Geometry check sheet. Reference: the model listing, model coordinates, mm. A direction names the side the tool comes from. Give positions to 0.01 mm unless a question says otherwise; leave off trailing zeros.
1. Release check for a two-part mould opening along Z. For faces 5 (the flat face through (22, 0, -12)), 6 (the flat face through (24, 0, -22)), 7 (the flat face through (9.6, -0.1, -2)), 8 (the flat face through (90, 0, 1)) record: +Z half, -Z half, draft (parallel to the pull), parting line (faces both ways), or undercut.
2. Go/stop test with flat-tipped pins: pin 1 Ø10 at (x, y) = (11.5, 1.5) entering from +Z; pin 2 Ø0.8 at (x, y) = (2.5, 2) entering from +Z; pin 3 Ø3.5 at (x, y) = (143.5, 0) entering from -Z. Record where each tip stops, or that it passes through.
3. Cross-section at A-A, the plane x = 143.5. State how many separate pieces and enclosed holes the cut face has, plus the area to 3 significant figures.
4. Material ranges on L1, parallel to Y at x = 12, z = -0.8; L2, parallel to Y at x = 38.5, z = 34.8; L3, parallel to X at y = -0.5, z = 17, recorded low to high.
5. Tool access check on faces 1 (the flat face through (2, 0, -18)), 2 (the cylindrical face through (6.254, -9.829, -16.143)), 3 (the cylindrical face through (6.2, -9.83, -7.81)), 4 (the flat face through (90, 0, 32)). Record the directions out of +Z, -Z, +X, -X, +Y, -Y that give a thin tool (end or side, any length) a straight path to the whole face; none if there is none.
from build123d import *

# Parameters (mm, degrees)
SKETCH_W          = 124
SKETCH_H          = 31
PAD_DEPTH         = 10
SKETCH001_R       = 2.1
POCKET_DEPTH      = 33.001
POCKET_DEPTH_BACK = 25.001
SKETCH002_R       = 4.5
POCKET001_DEPTH   = 33.001
FILLET_R          = 2
SKETCH003_R       = 1.6
POCKET002_DEPTH   = 4.001
FILLET001_R       = 0.6


with BuildPart() as part:
    # Sketch → Pad (new body, symmetric)
    with BuildSketch(Plane.XZ):
        Polygon((0, 0), (0, -22), (2, -22), (2, -14.6), (3.5, -14.6), (3.5, -18), (4.5, -18), (8.2, -14.6), (8.2, -9.4), (4.5, -6), (3.5, -6), (3.5, -9.4), (2, -9.4), (2, -2), (22, -2), (22, -22), (27, -22), (157, -5), (157, 0), (157, 36), (25, 36), align=None)
        with Locations((91, 16.5)):
            Rectangle(SKETCH_W, SKETCH_H, mode=Mode.SUBTRACT)
    extrude(amount=PAD_DEPTH, both=True)

    # Sketch001 (on Face14 of Pad) → Pocket (cut, two sides)
    with BuildSketch(Plane(origin=(0, 0, 3), x_dir=(1, 0, 0), z_dir=(0, 0, -1))) as pocket_sk:
        with Locations((12, 0)):
            Circle(SKETCH001_R)
    extrude(amount=-POCKET_DEPTH, mode=Mode.SUBTRACT)
    extrude(pocket_sk.sketch, amount=POCKET_DEPTH_BACK, mode=Mode.SUBTRACT)

    # Sketch002 (on Face14 of Pad) → Pocket001 (cut, through all)
    with BuildSketch(Plane(origin=(0, 0, 3), x_dir=(1, 0, 0), z_dir=(0, 0, -1))):
        with Locations((12, 0)):
            Circle(SKETCH002_R)
    extrude(amount=-POCKET001_DEPTH, mode=Mode.SUBTRACT)

    # Fillet
    fillet_edges = [part.edges().sort_by_distance(p)[0] for p in [
        (7.500022, -0.014101, 10.800032),
    ]]
    fillet(fillet_edges, radius=FILLET_R)

    # Sketch003 (on Face25 of Fillet) → Pocket002 (cut, through all)
    with BuildSketch(Plane(origin=(0, 0, 32), x_dir=(1, 0, 0), z_dir=(0, 0, -1))):
        with Locations((38.5, 0)):
            Circle(SKETCH003_R)
        with Locations((143.5, 0)):
            Circle(SKETCH003_R)
    extrude(amount=-POCKET002_DEPTH, mode=Mode.SUBTRACT)

    # Fillet001
    fillet001_edges = [part.edges().sort_by_distance(p)[0] for p in [
        (0, -10, -11),
        (1, -10, -22),
        (2, -10, -18.3),
        (2.75, -10, -14.6),
        (3.5, -10, -16.3),
        (4, -10, -18),
        (6.35, -10, -16.3),
        (8.2, -10, -12),
        (6.35, -10, -7.7),
        (4, -10, -6),
        (3.5, -10, -7.7),
        (2.75, -10, -9.4),
        (2, -10, -5.7),
        (12, -10, -2),
        (22, -10, -12),
        (24.5, -10, -22),
        (92, -10, -13.5),
        (157, -10, 15.5),
        (91, -10, 36),
        (12.5, -10, 18),
        (91, -10, 32),
        (153, -10, 16.5),
        (91, -10, 1),
        (29, -10, 16.5),
        (0, 10, -11),
        (1, 10, -22),
        (2, 10, -18.3),
        (2.75, 10, -14.6),
        (3.5, 10, -16.3),
        (4, 10, -18),
        (6.35, 10, -16.3),
        (8.2, 10, -12),
        (6.35, 10, -7.7),
        (4, 10, -6),
        (3.5, 10, -7.7),
        (2.75, 10, -9.4),
        (2, 10, -5.7),
        (12, 10, -2),
        (22, 10, -12),
        (24.5, 10, -22),
        (92, 10, -13.5),
        (157, 10, 15.5),
        (91, 10, 36),
        (12.5, 10, 18),
        (91, 10, 32),
        (153, 10, 16.5),
        (91, 10, 1),
        (29, 10, 16.5),
    ]]
    fillet(fillet001_edges, radius=FILLET001_R)


solid = part.part
Result:
1. face 5: draft
1. face 6: -Z half
1. face 7: undercut
1. face 8: undercut
2. pin 1: stops at z = 23.73
2. pin 2: stops at z = 4.18
2. pin 3: stops at z = -6.99
3. separate pieces: 3
3. enclosed holes: 0
3. area: 222 mm2
4. L1: y = -10 to -2.1, 2.1 to 10
4. L2: y = -10 to -1.6, 1.6 to 10
4. L3: x = 16.47 to 29, 153 to 157
5. face 1: -Z, +Y, -Y
5. face 2: -Z, -Y
5. face 3: -Y
5. face 4: +Y, -Y
